For this review, take the finished solid that the model builds, in its own axes (mm). Coordinates: 2 decimals unless noted, no trailing zeros. Order: outer loops, then holes, each group sorted by start corner. A loop starts at its lowest first (then second) coordinate and runs counter-clockwise, first axis right, second up. Notation, with made-up numbers: M 62.5,-27.75 L 119.5,-27.75 A22 cw 119.5,-2.75 Z; hole C 50.25,-7 d8. An arc over 180 degrees is marked long. Use CSV: the item, a comma, the result in double quotes.
```python
from build123d import *

# Parameters (mm, degrees)
F1_DEPTH = 50.4
F2_R     = 9.99999


# Not quite as in the source:
# - a fillet or chamfer is up to 0.001 mm smaller than in the source, because OpenCascade refuses the exact size


with BuildPart() as f1:
    # F0 (on Right) → F1 (new body, symmetric)
    with BuildSketch(Plane.YZ):
        with BuildLine():
            Line((-5, -5), (5, -5))
            Line((5, -5), (5, 5))
            ThreePointArc((5, 5), (-2.0710678119, 2.0710678119), (-5, -5))
        make_face()
    extrude(amount=F1_DEPTH, both=True)

    # F2 (radius 10 in the source; OpenCascade refuses exactly that, so slightly less here)
    f2_edges = [f1.edges().sort_by_distance(p)[0] for p in [
        (50.4, -2.071068, 2.071068),
        (-50.4, -2.071068, 2.071068),
    ]]
    fillet(f2_edges, radius=F2_R)


solid = f1.part
```
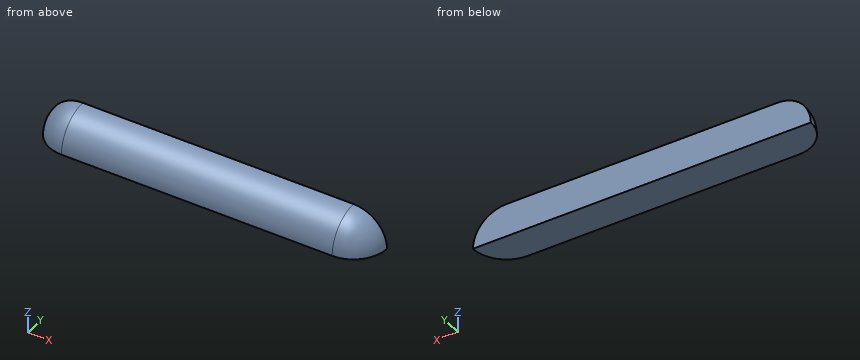
Item 1: Clearance check with flat-ended pins moving along their axes: pin 1 Ø1 at (x, z) = (40, -3) entering from -Y; pin 2 Ø1 at (y, z) = (2, 0) entering from +X; pin 3 Ø1 at (y, z) = (3, -1) entering from +X. State where each tip first meets the part, or that it passes through.
Solutions:
pin 1,"y = -4.89"
pin 2,"x = 48.86"
pin 3,"x = 49.58"
Item 2: Add section A-A on x = 29.5. State the section outline as (y, z) points, and give its area (3 significant figures).
Solutions:
outline,"M -5,-5 L 5,-5 L 5,5 A10 ccw Z"
area,"78.5 mm^2"
Item 3: To check wall thickness, follow line 1 along Y through (x, z) = (-14, 2.75); line 2 along Z through (x, y) = (27.5, 0.25); line 3 along Z through (x, y) = (33, 3.25). State the ranges of each line that lie inside material, in increasing order. Write a range as [from, to].
Solutions:
line 1,"[-1.32, 5]"
line 2,"[-5, 3.8]"
line 3,"[-5, 4.85]"
